Work out the finished part from the listing and answer in its coordinate system (mm). A direction names the side the tool comes from. Give positions to 0.01 mm unless a question says otherwise; leave off trailing zeros. Write each loop counter-clockwise with the first axis right and the second up, starting at its lowest first coordinate (ties: lowest second). Pieces come first, ordered by that corner, then holes. Notation, with made-up numbers: (-10.75, 44) - (26.25, 44) arc R34 ccw to (26.25, 82) - close; hole circle Ø9 at (-34.5, -11). An arc over 180 degrees is marked (long way). Write item = value, one per line.
from build123d import *

# Parameters (mm, degrees)
SKETCH1_R            = 35
BOSS_EXTRUDE1_DEPTH  = 9
SKETCH2_R            = 30
CUT_EXTRUDE1_DEPTH   = 3
SKETCH3_R            = 1.75
CUT_EXTRUDE2_DEPTH   = 51.309044912
SKETCH4_R            = 3.25
CUT_EXTRUDE3_DEPTH   = 3
BOSS_EXTRUDE3_START  = -9
BOSS_EXTRUDE3_DEPTH  = 9
SKETCH21_W           = 70
SKETCH21_H           = 6
BOSS_EXTRUDE8_DEPTH  = 6
SKETCH26_R           = 45
BOSS_EXTRUDE12_DEPTH = 6
CUT_EXTRUDE20_REACH  = 112.431
SKETCH27_R           = 1.75
SKETCH28_R           = 3.25
CUT_EXTRUDE21_DEPTH  = 3
CUT_EXTRUDE23_DEPTH  = 106.768615383


with BuildPart() as part:
    # Sketch1 → Boss-Extrude1 (new body)
    with BuildSketch(Plane(origin=(0, 0, 0), x_dir=(1, 0, 0), z_dir=(0, 1, 0))):
        with Locations(Location((0, 0, 0), (0, 0, 270))):
            Circle(SKETCH1_R)
    extrude(amount=BOSS_EXTRUDE1_DEPTH)

    # Sketch2 → Cut-Extrude1 (cut)
    with BuildSketch(Plane.XZ):
        with Locations(Location((0, 0, 0), (0, 0, 270))):
            Circle(SKETCH2_R)
    extrude(amount=-CUT_EXTRUDE1_DEPTH, mode=Mode.SUBTRACT)

    # Sketch3 → Cut-Extrude2 (cut, through all)
    with BuildSketch(Plane(origin=(0, 9, 0), x_dir=(1, 0, 0), z_dir=(0, 1, 0))):
        with Locations(Location((0, -25, 0), (0, 0, 270))):
            Circle(SKETCH3_R)
        with Locations(Location((-21.650635095, -12.5, 0), (0, 0, 270))):
            Circle(SKETCH3_R)
        with Locations(Location((-21.650635095, 12.5, 0), (0, 0, 270))):
            Circle(SKETCH3_R)
        with Locations(Location((0, 25, 0), (0, 0, 270))):
            Circle(SKETCH3_R)
        with Locations(Location((21.650635095, 12.5, 0), (0, 0, 270))):
            Circle(SKETCH3_R)
        with Locations(Location((21.650635095, -12.5, 0), (0, 0, 270))):
            Circle(SKETCH3_R)
    extrude(amount=-CUT_EXTRUDE2_DEPTH, mode=Mode.SUBTRACT)

    # Sketch4 → Cut-Extrude3 (cut)
    with BuildSketch(Plane(origin=(0, 9, 0), x_dir=(1, 0, 0), z_dir=(0, 1, 0))):
        with Locations(Location((0, 25, 0), (0, 0, 270))):
            Circle(SKETCH4_R)
        with Locations(Location((21.650635095, 12.5, 0), (0, 0, 270))):
            Circle(SKETCH4_R)
        with Locations(Location((21.650635095, -12.5, 0), (0, 0, 270))):
            Circle(SKETCH4_R)
        with Locations(Location((0, -25, 0), (0, 0, 270))):
            Circle(SKETCH4_R)
        with Locations(Location((-21.650635095, -12.5, 0), (0, 0, 270))):
            Circle(SKETCH4_R)
        with Locations(Location((-21.650635095, 12.5, 0), (0, 0, 270))):
            Circle(SKETCH4_R)
    extrude(amount=-CUT_EXTRUDE3_DEPTH, mode=Mode.SUBTRACT)

    # Sketch5 → Boss-Extrude3 (add)
    with BuildSketch(Plane(origin=(0, 9, 0), x_dir=(1, 0, 0), z_dir=(0, 1, 0)).offset(BOSS_EXTRUDE3_START)):
        with BuildLine():
            ThreePointArc((35, 0), (0, -35), (-35, 0))
            Line((-35, 0), (-35, -52))
            Line((-35, -52), (35, -52))
            Line((35, -52), (35, 0))
        make_face()
    extrude(amount=BOSS_EXTRUDE3_DEPTH)

    # Sketch21 → Boss-Extrude8 (add)
    with BuildSketch(Plane.XZ):
        with Locations((0, 49)):
            Rectangle(SKETCH21_W, SKETCH21_H)
    extrude(amount=BOSS_EXTRUDE8_DEPTH)

    # Sketch26 → Boss-Extrude12 (add)
    with BuildSketch(Plane.XY.offset(52)):
        with Locations((0, -6)):
            Circle(SKETCH26_R)
    extrude(amount=-BOSS_EXTRUDE12_DEPTH)

    # Sketch27 → Cut-Extrude20 (cut, up to next)
    with BuildSketch(Plane.XY.offset(52), mode=Mode.PRIVATE) as cut_extrude20_sk1:
        with Locations((0, -46.031695342)):
            Circle(SKETCH27_R)
    cut_extrude20_tool1 = extrude(cut_extrude20_sk1.sketch, amount=-CUT_EXTRUDE20_REACH, mode=Mode.PRIVATE) & part.part
    # Sketch27 → Cut-Extrude20 (cut, up to next)
    with BuildSketch(Plane.XY.offset(52), mode=Mode.PRIVATE) as cut_extrude20_sk2:
        with Locations((-20.015847671, -40.668465123)):
            Circle(SKETCH27_R)
    cut_extrude20_tool2 = extrude(cut_extrude20_sk2.sketch, amount=-CUT_EXTRUDE20_REACH, mode=Mode.PRIVATE) & part.part
    # Sketch27 → Cut-Extrude20 (cut, up to next)
    with BuildSketch(Plane.XY.offset(52), mode=Mode.PRIVATE) as cut_extrude20_sk3:
        with Locations((-34.668465123, -26.015847671)):
            Circle(SKETCH27_R)
    cut_extrude20_tool3 = extrude(cut_extrude20_sk3.sketch, amount=-CUT_EXTRUDE20_REACH, mode=Mode.PRIVATE) & part.part
    # Sketch27 → Cut-Extrude20 (cut, up to next)
    with BuildSketch(Plane.XY.offset(52), mode=Mode.PRIVATE) as cut_extrude20_sk4:
        with Locations((-40.031695342, -6)):
            Circle(SKETCH27_R)
    cut_extrude20_tool4 = extrude(cut_extrude20_sk4.sketch, amount=-CUT_EXTRUDE20_REACH, mode=Mode.PRIVATE) & part.part
    # Sketch27 → Cut-Extrude20 (cut, up to next)
    with BuildSketch(Plane.XY.offset(52), mode=Mode.PRIVATE) as cut_extrude20_sk5:
        with Locations((-34.668465123, 14.015847671)):
            Circle(SKETCH27_R)
    cut_extrude20_tool5 = extrude(cut_extrude20_sk5.sketch, amount=-CUT_EXTRUDE20_REACH, mode=Mode.PRIVATE) & part.part
    # Sketch27 → Cut-Extrude20 (cut, up to next)
    with BuildSketch(Plane.XY.offset(52), mode=Mode.PRIVATE) as cut_extrude20_sk6:
        with Locations((-20.015847671, 28.668465123)):
            Circle(SKETCH27_R)
    cut_extrude20_tool6 = extrude(cut_extrude20_sk6.sketch, amount=-CUT_EXTRUDE20_REACH, mode=Mode.PRIVATE) & part.part
    # Sketch27 → Cut-Extrude20 (cut, up to next)
    with BuildSketch(Plane.XY.offset(52), mode=Mode.PRIVATE) as cut_extrude20_sk7:
        with Locations((0, 34.031695342)):
            Circle(SKETCH27_R)
    cut_extrude20_tool7 = extrude(cut_extrude20_sk7.sketch, amount=-CUT_EXTRUDE20_REACH, mode=Mode.PRIVATE) & part.part
    # Sketch27 → Cut-Extrude20 (cut, up to next)
    with BuildSketch(Plane.XY.offset(52), mode=Mode.PRIVATE) as cut_extrude20_sk8:
        with Locations((20.015847671, 28.668465123)):
            Circle(SKETCH27_R)
    cut_extrude20_tool8 = extrude(cut_extrude20_sk8.sketch, amount=-CUT_EXTRUDE20_REACH, mode=Mode.PRIVATE) & part.part
    # Sketch27 → Cut-Extrude20 (cut, up to next)
    with BuildSketch(Plane.XY.offset(52), mode=Mode.PRIVATE) as cut_extrude20_sk9:
        with Locations((34.668465123, 14.015847671)):
            Circle(SKETCH27_R)
    cut_extrude20_tool9 = extrude(cut_extrude20_sk9.sketch, amount=-CUT_EXTRUDE20_REACH, mode=Mode.PRIVATE) & part.part
    # Sketch27 → Cut-Extrude20 (cut, up to next)
    with BuildSketch(Plane.XY.offset(52), mode=Mode.PRIVATE) as cut_extrude20_sk10:
        with Locations((40.031695342, -6)):
            Circle(SKETCH27_R)
    cut_extrude20_tool10 = extrude(cut_extrude20_sk10.sketch, amount=-CUT_EXTRUDE20_REACH, mode=Mode.PRIVATE) & part.part
    # Sketch27 → Cut-Extrude20 (cut, up to next)
    with BuildSketch(Plane.XY.offset(52), mode=Mode.PRIVATE) as cut_extrude20_sk11:
        with Locations((34.668465123, -26.015847671)):
            Circle(SKETCH27_R)
    cut_extrude20_tool11 = extrude(cut_extrude20_sk11.sketch, amount=-CUT_EXTRUDE20_REACH, mode=Mode.PRIVATE) & part.part
    # Sketch27 → Cut-Extrude20 (cut, up to next)
    with BuildSketch(Plane.XY.offset(52), mode=Mode.PRIVATE) as cut_extrude20_sk12:
        with Locations((20.015847671, -40.668465123)):
            Circle(SKETCH27_R)
    cut_extrude20_tool12 = extrude(cut_extrude20_sk12.sketch, amount=-CUT_EXTRUDE20_REACH, mode=Mode.PRIVATE) & part.part
    add(cut_extrude20_tool1.solids().sort_by_distance((0, -46.031695, 52))[0], mode=Mode.SUBTRACT)
    add(cut_extrude20_tool2.solids().sort_by_distance((-20.015848, -40.668465, 52))[0], mode=Mode.SUBTRACT)
    add(cut_extrude20_tool3.solids().sort_by_distance((-34.668465, -26.015848, 52))[0], mode=Mode.SUBTRACT)
    add(cut_extrude20_tool4.solids().sort_by_distance((-40.031695, -6, 52))[0], mode=Mode.SUBTRACT)
    add(cut_extrude20_tool5.solids().sort_by_distance((-34.668465, 14.015848, 52))[0], mode=Mode.SUBTRACT)
    add(cut_extrude20_tool6.solids().sort_by_distance((-20.015848, 28.668465, 52))[0], mode=Mode.SUBTRACT)
    add(cut_extrude20_tool7.solids().sort_by_distance((0, 34.031695, 52))[0], mode=Mode.SUBTRACT)
    add(cut_extrude20_tool8.solids().sort_by_distance((20.015848, 28.668465, 52))[0], mode=Mode.SUBTRACT)
    add(cut_extrude20_tool9.solids().sort_by_distance((34.668465, 14.015848, 52))[0], mode=Mode.SUBTRACT)
    add(cut_extrude20_tool10.solids().sort_by_distance((40.031695, -6, 52))[0], mode=Mode.SUBTRACT)
    add(cut_extrude20_tool11.solids().sort_by_distance((34.668465, -26.015848, 52))[0], mode=Mode.SUBTRACT)
    add(cut_extrude20_tool12.solids().sort_by_distance((20.015848, -40.668465, 52))[0], mode=Mode.SUBTRACT)

    # Sketch28 → Cut-Extrude21 (cut)
    with BuildSketch(Plane(origin=(0, 0, 46), x_dir=(-1, 0, 0), z_dir=(0, 0, -1))):
        with Locations((0, -46.031695342)):
            Circle(SKETCH28_R)
        with Locations((-20, -40.672711494)):
            Circle(SKETCH28_R)
        with Locations((-34.641016151, -26.031695342)):
            Circle(SKETCH28_R)
        with Locations((-40, -6.031695342)):
            Circle(SKETCH28_R)
        with Locations((-34.641016151, 13.968304658)):
            Circle(SKETCH28_R)
        with Locations((-20, 28.609320809)):
            Circle(SKETCH28_R)
        with Locations((0, 33.968304658)):
            Circle(SKETCH28_R)
        with Locations((20, 28.609320809)):
            Circle(SKETCH28_R)
        with Locations((34.641016151, 13.968304658)):
            Circle(SKETCH28_R)
        with Locations((40, -6.031695342)):
            Circle(SKETCH28_R)
        with Locations((34.641016151, -26.031695342)):
            Circle(SKETCH28_R)
        with Locations((20, -40.672711494)):
            Circle(SKETCH28_R)
    extrude(amount=-CUT_EXTRUDE21_DEPTH, mode=Mode.SUBTRACT)

    # Sketch30 → Cut-Extrude23 (cut, through all)
    with BuildSketch(Plane(origin=(0, 0, 46), x_dir=(-1, 0, 0), z_dir=(0, 0, -1))):
        with BuildLine():
            Line((-3, -10.325026058), (-3, -40.871191548))
            ThreePointArc((-3, -40.871191548), (-14.085565968, -38.040549798), (-23.665962091, -31.786086138))
            Line((-23.665962091, -31.786086138), (-3, -10.325026058))
        make_face()
        with BuildLine():
            Line((3, -10.325026058), (3, -40.871191548))
            ThreePointArc((3, -40.871191548), (14.085565968, -38.040549798), (23.665962091, -31.786086138))
            Line((23.665962091, -31.786086138), (3, -10.325026058))
        make_face()
        with BuildLine():
            Line((-7.164790753, -6), (-35, -6))
            ThreePointArc((-35, -6), (-33.132555391, -17.279794913), (-27.729498669, -27.355910272))
            Line((-27.729498669, -27.355910272), (-7.164790753, -6))
        make_face()
        with BuildLine():
            Line((7.164790753, -6), (35, -6))
            ThreePointArc((35, -6), (33.132555391, -17.279794913), (27.729498669, -27.355910272))
            Line((27.729498669, -27.355910272), (7.164790753, -6))
        make_face()
        with BuildLine():
            Line((-24.748737342, 18.748737342), (-17.67766953, 11.67766953))
            Line((-17.67766953, 11.67766953), (17.67766953, 11.67766953))
            Line((17.67766953, 11.67766953), (24.748737342, 18.748737342))
            ThreePointArc((24.748737342, 18.748737342), (0, 29), (-24.748737342, 18.748737342))
        make_face()
    extrude(amount=-CUT_EXTRUDE23_DEPTH, mode=Mode.SUBTRACT)


solid = part.part
1. Find section B-B, the plane y = -17.5. Give the vertices of the cut face in (x, z), then the cut area to 3 significant figures.
Solution:
outline = (-43.51, 46) - (-33.06, 46) - (-33.06, 52) - (-43.51, 52) - close; (-18.24, 46) - (-9.91, 46) - (-9.91, 52) - (-18.24, 52) - close; (-3, 46) - (3, 46) - (3, 52) - (-3, 52) - close; (9.91, 46) - (18.24, 46) - (18.24, 52) - (9.91, 52) - close; (33.06, 46) - (43.51, 46) - (43.51, 52) - (33.06, 52) - close
area = 261 mm^2
2. Find section A-A, the plane z = 25. Give the vertices of the cut face in (x, y).
Solution:
outline = (-35, 0) - (-16.58, 0) - (-16.58, 3) - (-1.75, 3) - (-1.75, 6) - (-3.25, 6) - (-3.25, 9) - (-35, 9) - close; (1.75, 3) - (16.58, 3) - (16.58, 0) - (35, 0) - (35, 9) - (3.25, 9) - (3.25, 6) - (1.75, 6) - close
3. Find section C-C, the plane x = 40. Give the vertices of the cut face in (y, z), then the cut area to 3 significant figures.
Solution:
outline = (-26.62, 46) - (-9.28, 46) - (-9.28, 49) - (-7.75, 49) - (-7.75, 52) - (-26.62, 52) - close; (-4.25, 49) - (-2.78, 49) - (-2.78, 46) - (14.62, 46) - (14.62, 52) - (-4.25, 52) - close
area = 217 mm^2
4. Straight lines are drawn through the part: line 1 (X direction, y = 8.25, z = 12.5); line 2 (Y direction, x = -21, z = -1); line 3 (Z direction, x = -33, y = -22.5). For each, find the intervals that lie inside material, in ascending order.
Solution:
line_1 = -35 to -24.9, -18.4 to 18.4, 24.9 to 35
line_2 = 3 to 9
line_3 = 46 to 52
5. For a pull along Y with two mould halves and no side action, classify faces 1 (the cylindrical face through (20.957, -39.193, 50.521)), 2 (the flat face through (-23, 6, 14)), 3 (the cylindrical face through (0.77, 4.44, -34.99)) as pulls with the +Y half, pulls with the -Y half, needs draft (parallel to the pull), parting line crosses it, or undercut.
Solution:
face_1 = undercut
face_2 = pulls with the +Y half
face_3 = needs draft
6. A tool of negligible diameter and unlimited length cuts with its end or side. For faces 4 (the cylindrical face through (20.1, 4.52, 13.31)), 5 (the cylindrical face through (0, 29, 49)), 6 (the flat face through (-1.4, 6, 26.4)), 7 (the cylindrical face through (22.58, -42.65, 47.48)), from which of +Z, -Z, +X, -X, +Y, -Y can it reach the whole face along a straight path? Write none if from no direction.
Solution:
face_4 = +Y, -Y
face_5 = +Z, -Z
face_6 = +Y
face_7 = -Z
7. Given pin 1 (1 mm diameter, centred on x = 4.5, y = -8.5, fed in from -Z); pin 2 (2 mm diameter, centred on x = -20.02, y = -40.67, fed in from +Z); pin 3 (3 mm diameter, centred on x = 22, z = 12, fed in from +Y); pin 4 (5.5 mm diameter, centred on x = -34.67, y = 14.02, fed in from -Z), each flat-ended and moving along its own axis, determine where each tip first touches the part or whether it passes through.
Solution:
pin_1 = 46
pin_2 = through
pin_3 = 6
pin_4 = 49
8. Find section D-D, the plane z = -12.5. Give the vertices of the cut face in (x, y), then the cut area to 3 significant figures.
Solution:
outline = (-32.69, 0) - (-27.27, 0) - (-27.27, 3) - (-23.4, 3) - (-23.4, 6) - (-24.9, 6) - (-24.9, 9) - (-32.69, 9) - close; (-19.9, 3) - (19.9, 3) - (19.9, 6) - (18.4, 6) - (18.4, 9) - (-18.4, 9) - (-18.4, 6) - (-19.9, 6) - close; (23.4, 3) - (27.27, 3) - (27.27, 0) - (32.69, 0) - (32.69, 9) - (24.9, 9) - (24.9, 6) - (23.4, 6) - close
area = 365 mm^2
